Read the model definition and answer for the solid it produces. Units are mm, in the model's axes. A direction names the side the tool comes from. Round coordinates to 2 decimals unless told otherwise and drop trailing zeros. Order: outer loops, then holes, each group sorted by start corner. A loop starts at its lowest first (then second) coordinate and runs counter-clockwise, first axis right, second up. Notation, with made-up numbers: (-8, 42.5) -> (-2, 42.5) arc R14 cw to (-2, 59.5) -> close; hole circle Ø5 at (-33.5, 65). An arc over 180 degrees is marked (long way). Answer as a JSON object with one key per item and string values. Group by question number.
Item 1: Consider probe 1 along Y at (x, z) = (26.5, 4.5); probe 2 along Z at (x, y) = (-12, -5.25); probe 3 along X at (y, z) = (-0.5, 0.75). Determine where each line is inside the solid, lowest interval first. Write a range as from..to.
Item 2: Section B-B, the plane y = 0 is taken. Write down the section's boundary in (x, z).
Item 3: Section A-A, the plane z = 5 is taken. Write down the section's boundary in (x, y), plus the area to 3 significant figures.
Item 4: Section D-D, the plane z = 1.75 is taken. Write down the section's boundary in (x, y), plus the area to 3 significant figures.
Item 5: For faces 5 (the cylindrical face through (19.1, 4.43, 4.73)), 6 (the flat face through (0, 0, 3)), 7 (the cylindrical face through (19.07, -4.4, 4.73)), determine the directions among +Z, -Z, +X, -X, +Y, -Y from which every point of the face is accessible in a straight line to the end or side of a thin tool.
Item 6: Given P1, Ø1.8, axis at x = 24, z = 4, coming from the +Y side; P2, Ø1.8, axis at y = 0, z = 5.5, coming from the +X side; P3, Ø3, axis at x = 24.5, z = 5, coming from the -Y side, each flat-ended and moving along its own axis, determine where each tip first touches the part or whether it passes through.
Item 7: The mould has two halves that part along Y. Classify faces 1 (the flat face through (18.5, 0, 5)), 2 (the cylindrical face through (29.93, 4.4, 4.73)), 3 (the cylindrical face through (29.84, 1.05, 3.3)), 4 (the cylindrical face through (-23.16, 1.05, 3.2)): pulls with the +Y half, pulls with the -Y half, needs draft (parallel to the pull), parting line crosses it, or undercut.
Item 8: Section C-C, the plane x = 26.5 is taken. Write down the section's boundary in (y, z), plus the area to 3 significant figures.
from build123d import *

# Parameters (mm, degrees)
F0_W     = 67
F0_H     = 16
F0_R     = 3.5
F1_DEPTH = 3
F3_DEPTH = 3.5
F4_R     = 3.5
F5_DEPTH = 6.501
F6_R     = 3


with BuildPart() as f1:
    # F0 (on Top) → F1 (new body)
    with BuildSketch(Plane.XY):
        Rectangle(F0_W, F0_H)
        with Locations((-26.5, 0)):
            Circle(F0_R, mode=Mode.SUBTRACT)
        with Locations((26.5, 0)):
            Circle(F0_R, mode=Mode.SUBTRACT)
    extrude(amount=F1_DEPTH)

    # F2 (on face) → F3 (join)
    with BuildSketch(Plane.XY.offset(3)):
        with BuildLine():
            Line((20.5, -5), (28.5, -5))
            ThreePointArc((28.5, -5), (29.914214, -4.414214), (30.5, -3))
            Line((30.5, -3), (30.5, 3))
            ThreePointArc((30.5, 3), (29.914214, 4.414214), (28.5, 5))
            Line((28.5, 5), (20.5, 5))
            ThreePointArc((20.5, 5), (19.085786, 4.414214), (18.5, 3))
            Line((18.5, 3), (18.5, -3))
            ThreePointArc((18.5, -3), (19.085786, -4.414214), (20.5, -5))
        make_face()
        with BuildLine():
            Line((-28.5, -5), (-20.5, -5))
            ThreePointArc((-20.5, -5), (-19.085786, -4.414214), (-18.5, -3))
            Line((-18.5, -3), (-18.5, 3))
            ThreePointArc((-18.5, 3), (-19.085786, 4.414214), (-20.5, 5))
            Line((-20.5, 5), (-28.5, 5))
            ThreePointArc((-28.5, 5), (-29.914214, 4.414214), (-30.5, 3))
            Line((-30.5, 3), (-30.5, -3))
            ThreePointArc((-30.5, -3), (-29.914214, -4.414214), (-28.5, -5))
        make_face()
    extrude(amount=F3_DEPTH)

    # F4 (on face) → F5 (cut, through all)
    with BuildSketch(Plane.XY.offset(6.5)):
        with Locations((26.5, 0)):
            Circle(F4_R)
        with Locations((-26.5, 0)):
            Circle(F4_R)
    extrude(amount=-F5_DEPTH, mode=Mode.SUBTRACT)

    # F6
    f6_edges = [f1.edges().sort_by_distance(p)[0] for p in [
        (-33.5, 8, 1.5),
        (33.5, 8, 1.5),
        (33.5, -8, 1.5),
        (-33.5, -8, 1.5),
    ]]
    fillet(f6_edges, radius=F6_R)


solid = f1.part
Values found:
{
 "1": {"probe 1": "-5..-3.5, 3.5..5", "probe 2": "0..3", "probe 3": "-33.5..-29.96, -23.04..23.04, 29.96..33.5"},
 "2": {"outline": "(-33.5, 0) -> (-30, 0) -> (-30, 6.5) -> (-30.5, 6.5) -> (-30.5, 3) -> (-33.5, 3) -> close; (-23, 0) -> (23, 0) -> (23, 6.5) -> (18.5, 6.5) -> (18.5, 3) -> (-18.5, 3) -> (-18.5, 6.5) -> (-23, 6.5) -> close; (30, 0) -> (33.5, 0) -> (33.5, 3) -> (30.5, 3) -> (30.5, 6.5) -> (30, 6.5) -> close"},
 "3": {"outline": "(-30.5, -3) arc R2 ccw to (-28.5, -5) -> (-20.5, -5) arc R2 ccw to (-18.5, -3) -> (-18.5, 3) arc R2 ccw to (-20.5, 5) -> (-28.5, 5) arc R2 ccw to (-30.5, 3) -> close; (18.5, -3) arc R2 ccw to (20.5, -5) -> (28.5, -5) arc R2 ccw to (30.5, -3) -> (30.5, 3) arc R2 ccw to (28.5, 5) -> (20.5, 5) arc R2 ccw to (18.5, 3) -> close; hole circle Ø7 at (-26.5, 0); hole circle Ø7 at (26.5, 0)", "area": "156 mm2"},
 "4": {"outline": "(-33.5, -5) arc R3 ccw to (-30.5, -8) -> (30.5, -8) arc R3 ccw to (33.5, -5) -> (33.5, 5) arc R3 ccw to (30.5, 8) -> (-30.5, 8) arc R3 ccw to (-33.5, 5) -> close; hole circle Ø7 at (-26.5, 0); hole circle Ø7 at (26.5, 0)", "area": "987 mm2"},
 "5": {"face 5": "+Z, +Y", "face 6": "+Z", "face 7": "+Z, -Y"},
 "6": {"P1": "y = 5", "P2": "x = 30.5", "P3": "y = -5"},
 "7": {"face 1": "needs draft", "face 2": "pulls with the +Y half", "face 3": "undercut", "face 4": "undercut"},
 "8": {"outline": "(-8, 0) -> (-3.5, 0) -> (-3.5, 6.5) -> (-5, 6.5) -> (-5, 3) -> (-8, 3) -> close; (3.5, 0) -> (8, 0) -> (8, 3) -> (5, 3) -> (5, 6.5) -> (3.5, 6.5) -> close", "area": "37.5 mm2"}
}
